Build history of the part. All positions in model axes, mm. Face numbers are marked on the shaded views. Coordinates: 2 decimals unless noted, no trailing zeros. Loops run counter-clockwise (first coordinate to the right, second up) from the corner with the lowest first, then second, coordinate; pieces in that order, holes last.
Item 1: Drill centre lines: line 1 along X through (y, z) = (-381, 84); line 2 along X through (y, z) = (-574.5, 114.5); line 3 along Y through (x, z) = (407.5, 12.5). Where is each one in solid material? Low to high.
Item 2: Flat gauge pins, fed straight in: pin 1 (10 mm diameter, centred on x = 405.5, y = -254, fed in from +Z); pin 2 (16 mm diameter, centred on x = 442.5, z = 92, fed in from +Y); pin 3 (10 mm diameter, centred on y = -473, z = 6, fed in from +X); pin 4 (1.5 mm diameter, centred on y = -602, z = 20, fed in from -X). Where does each tip first touch, or does it go through?
Item 3: Cut at A-A (y = -604.5). List the corners of the cut face in (x, z).
Item 4: Mould opens along Y. For the marked faces 1 and 2 say: released by +Y, released by -Y, zero draft, split by the parting line, or undercut.
Item 5: Cut at C-C (y = -292.5). Count the separate pieces of the cut face and the enclosed holes in it, and give its area (3 significant figures).
Item 6: Cut at B-B (x = 410). List the corners of the cut face in (y, z).
from build123d import *

# Parameters (mm, degrees)
F0_W     = 260
F0_H     = 20
F0_W_2   = 20
F0_H_2   = 360
F1_DEPTH = 20
F2_W     = 20
F2_H     = 20
F2_H_2   = 150
F3_DEPTH = 70
F5_D     = 40
F6_R     = 75


with BuildPart() as f1:
    # F0 (on Top) → F1 (new body)
    with BuildSketch(Plane.XY):
        Polygon((600, 0), (0, 0), (0, -20), (20, -20), (200, -20), (220, -20), (380, -20), (400, -20), (580, -20), (600, -20), align=None)
        Polygon((20, -20), (0, -20), (0, -400), (20, -400), (20, -380), align=None)
        Polygon((600, -400), (600, -20), (580, -20), (580, -380), (580, -400), align=None)
        Polygon((20, -400), (0, -400), (150, -585), (150, -560.333333), align=None)
        Polygon((450, -585), (600, -400), (580, -400), (450, -560.333333), align=None)
        Polygon((150, -560.333333), (150, -585), (150, -700), (170, -700), (170, -570), (170, -550), (170, -400), (150, -400), align=None)
        Polygon((450, -700), (450, -585), (450, -560.333333), (450, -400), (430, -400), (430, -550), (430, -570), (430, -700), align=None)
        with Locations((300, -560)):
            Rectangle(F0_W, F0_H)
        with Locations((390, -200)):
            Rectangle(F0_W_2, F0_H_2)
        Polygon((200, -380), (20, -380), (20, -400), (150, -400), (170, -400), (430, -400), (450, -400), (580, -400), (580, -380), (400, -380), (380, -380), (220, -380), align=None)
        with Locations((210, -200)):
            Rectangle(F0_W_2, F0_H_2)
    extrude(amount=F1_DEPTH)

    # F2 (on face) → F3 (join)
    with BuildSketch(Plane.XY.offset(20)):
        with Locations((10, -10)):
            Rectangle(F2_W, F2_H)
        with Locations((590, -10)):
            Rectangle(F2_W, F2_H)
        with Locations((590, -390)):
            Rectangle(F2_W, F2_H)
        with Locations((10, -390)):
            Rectangle(F2_W, F2_H)
        with Locations((160, -625)):
            Rectangle(F2_W, F2_H_2)
        with Locations((440, -625)):
            Rectangle(F2_W, F2_H_2)
        with Locations((300, -390)):
            Rectangle(F2_W, F2_H)
        with Locations((300, -10)):
            Rectangle(F2_W, F2_H)
    extrude(amount=F3_DEPTH)

    # F5 (through all)
    with Locations(Plane.YZ.offset(450)):
        with Locations((-650, 90)):
            Hole(F5_D / 2)

    # F6
    f6_edges = [f1.edges().sort_by_distance(p)[0] for p in [
        (160, -700, 0),
        (440, -700, 0),
    ]]
    fillet(f6_edges, radius=F6_R)

    # F7: F1 across face


with BuildPart() as f1_1:
    add(f1.part)
    add(f1.part.mirror(Plane(origin=(160, -590, 90), x_dir=(1, 0, 0), z_dir=(0, 0, 1))))


solid = f1_1.part
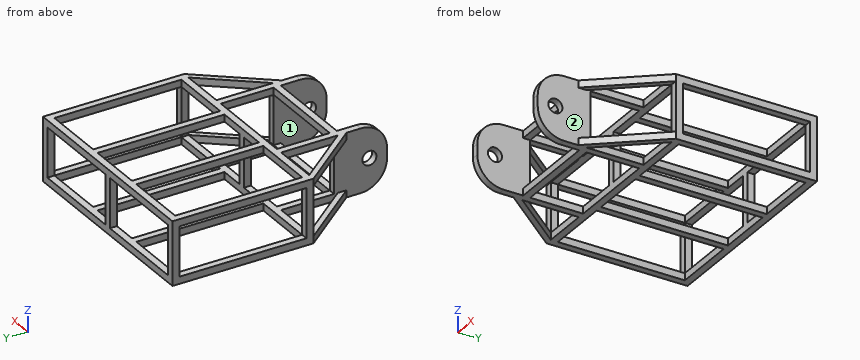
Filled sheet:
1. line 1: x = 0 to 20, 290 to 310, 580 to 600
1. line 2: x = 150 to 170, 430 to 450
1. line 3: y = -570 to -550, -400 to -380, -20 to 0
2. pin 1: passes through
2. pin 2: stops at y = -550
2. pin 3: stops at x = 544.86
2. pin 4: stops at x = 150
3. outline: (150, 0) - (170, 0) - (170, 180) - (150, 180) - close; (430, 0) - (450, 0) - (450, 180) - (430, 180) - close
4. face 1: zero draft
4. face 2: undercut
5. separate pieces: 8
5. enclosed holes: 0
5. area: 3,200 mm2
6. outline: (-570, 0) - (-550, 0) - (-550, 20) - (-570, 20) - close; (-570, 160) - (-550, 160) - (-550, 180) - (-570, 180) - close; (-400, 0) - (-380, 0) - (-380, 20) - (-400, 20) - close; (-400, 160) - (-380, 160) - (-380, 180) - (-400, 180) - close; (-20, 0) - (0, 0) - (0, 20) - (-20, 20) - close; (-20, 160) - (0, 160) - (0, 180) - (-20, 180) - close
